Can you work these out from the drawing? Everything is in mm from the part's minimum corner. A direction names the side the tool comes from. Give positions to 0.01 mm unless a question says otherwise; leave off trailing zeros. Write each loop counter-clockwise with the first axis right and the second up, starting at its lowest first coordinate (ties: lowest second). Pieces come first, ordered by that corner, then holes. Notation, with made-up numbers: (19, 43) - (30, 43) arc R22 cw to (30, 63) - close; hole circle Ø8 at (77.5, 75). An arc over 180 degrees is marked (long way). Return JSON: item names as keys, results as strings. Group by question number.
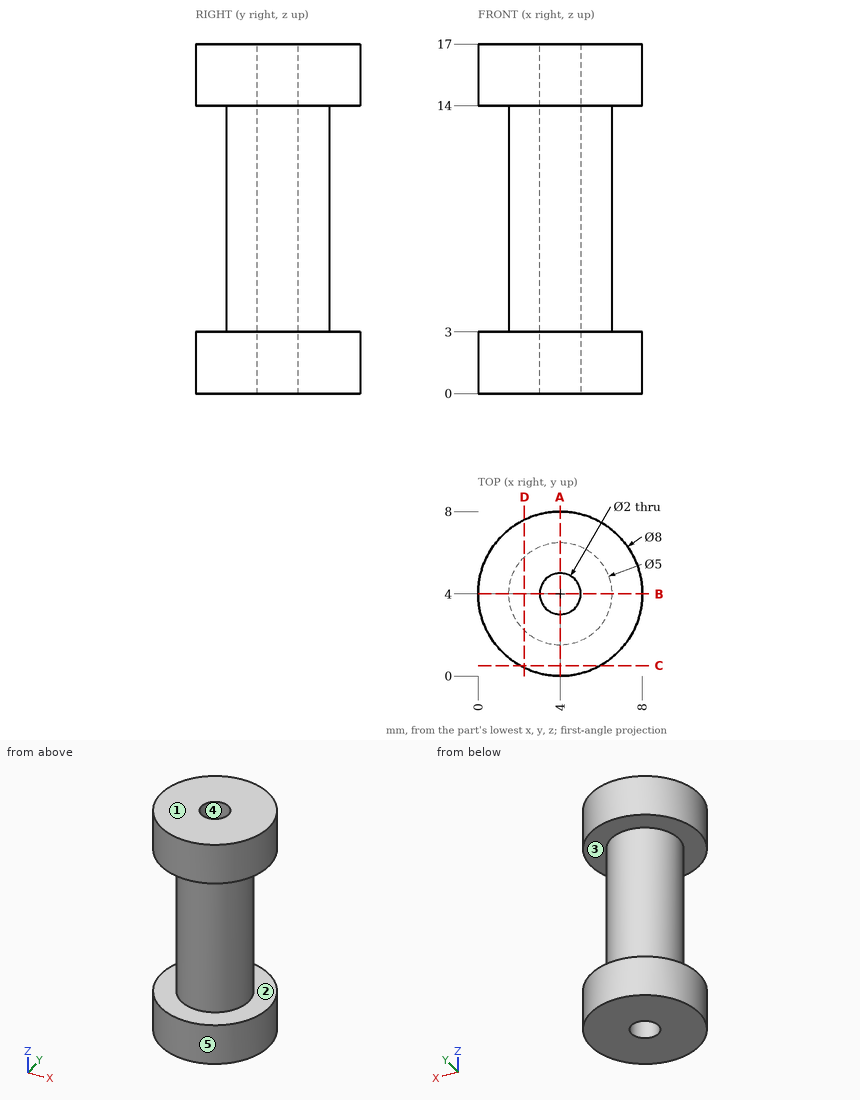
1) Imagine slicing it at C-C, the plane y = 0.5. Write out the boundary of the cut face in (x, z), and give its area (3 significant figures).
2) I need wall thicknesses on line 1 along Z through (x, y) = (1, 5.75); line 2 along Y through (x, z) = (4, 9); line 3 along Y through (x, z) = (3.5, 3.5). Which ranges of each line are inside material? Lowest first, please.
3) We'd pull the mould along Y, two halves only. Please class the marked faces 3, 4 and 5: pulls with the +Y half, pulls with the -Y half, needs draft (parallel to the pull), parting line crosses it, or undercut.
4) Imagine slicing it at D-D, the plane x = 2.25. Write out the boundary of the cut face in (y, z).
5) Imagine slicing it at A-A, the plane x = 4. Write out the boundary of the cut face in (y, z).
6) Will these pins go through, and if not, where does the flat tip stop? pin 1 Ø1.6 at (x, y) = (4, 4) entering from -Z; pin 2 Ø1.5 at (x, z) = (5.5, 6) entering from -Y; pin 3 Ø1 at (y, z) = (1.5, 6.5) entering from -X.
7) On a 3-axis mill with a long thin cutter (end or side, diameter ignored), from which of +Z, -Z, +X, -X, +Y, -Y can I reach the whole of each face in a straight line? I mean the marked faces 1 and 2. Say none if no direction works.
Resolved:
{
 "1": {"outline": "(2.06, 0) - (5.94, 0) - (5.94, 3) - (2.06, 3) - close; (2.06, 14) - (5.94, 14) - (5.94, 17) - (2.06, 17) - close", "area": "23.2 mm^2"},
 "2": {"line 1": "0 to 3, 14 to 17", "line 2": "1.5 to 3, 5 to 6.5", "line 3": "1.55 to 3.13, 4.87 to 6.45"},
 "3": {"face 3": "needs draft", "face 4": "undercut", "face 5": "parting line crosses it"},
 "4": {"outline": "(0.4, 0) - (7.6, 0) - (7.6, 3) - (5.79, 3) - (5.79, 14) - (7.6, 14) - (7.6, 17) - (0.4, 17) - (0.4, 14) - (2.21, 14) - (2.21, 3) - (0.4, 3) - close"},
 "5": {"outline": "(0, 0) - (3, 0) - (3, 17) - (0, 17) - (0, 14) - (1.5, 14) - (1.5, 3) - (0, 3) - close; (5, 0) - (8, 0) - (8, 3) - (6.5, 3) - (6.5, 14) - (8, 14) - (8, 17) - (5, 17) - close"},
 "6": {"pin 1": "through", "pin 2": "y = 1.62", "pin 3": "x = 2.5"},
 "7": {"face 1": "+Z, +X, -X, +Y, -Y", "face 2": "none"}
}
